Geometry check sheet. Reference: the model listing, model coordinates, mm. Face numbers are marked on the shaded views. A direction names the side the tool comes from. Give positions to 0.01 mm unless a question says otherwise; leave off trailing zeros. Loops run counter-clockwise (first coordinate to the right, second up) from the corner with the lowest first, then second, coordinate; pieces in that order, holes last.
1. Material ranges on L1, parallel to X at y = 2.7, z = -53 (3 decimals); L2, parallel to X at y = 1.35, z = -52; L3, parallel to Z at x = 7, y = 1.5, recorded low to high.
2. Cross-section at D-D, the plane x = -20. Record the cut outline in (y, z).
3. Cross-section at C-C, the plane x = -49. Record the cut outline in (y, z), plus the area to 3 significant figures.
4. Cross-section at A-A, the plane z = -59.5. Record the cut outline in (x, y).
5. Cross-section at B-B, the plane z = -22. Record the cut outline in (x, y), plus the area to 3 significant figures.
6. Tool access check on the marked faces 1 and 2. Record the directions out of +Z, -Z, +X, -X, +Y, -Y that give a thin tool (end or side, any length) a straight path to the whole face; none if there is none.
7. Go/stop test with flat-tipped pins: pin 1 Ø0.6 at (y, z) = (0.5, -8) entering from -X; pin 2 Ø1 at (x, y) = (-86.5, 0.5) entering from -Z; pin 3 Ø1 at (x, z) = (-79.5, -15.5) entering from +Y. Record where each tip stops, or that it passes through.
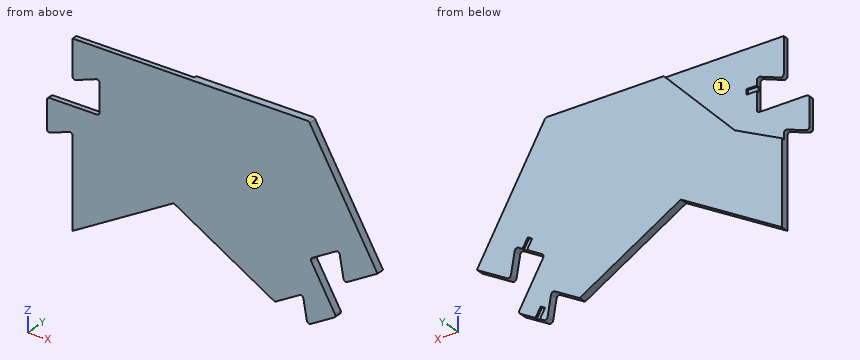
from build123d import *

# Parameters (mm, degrees)
P_IDAT_VYSUNUT_M1_DEPTH  = 3
P_IDAT_VYSUNUT_M2_DEPTH  = 2
ZAOBLIT1_R               = 1
SKICA3_W                 = 4
SKICA3_H                 = 2
ODEBRAT_VYSUNUT_M1_DEPTH = 0.8
ODEBRAT_VYSUNUT_M2_DEPTH = 0.8


with BuildPart() as part:
    # Skica1 → P_idat vysunut_m1 (new body)
    with BuildSketch(Plane(origin=(0, 0, 0), x_dir=(1, 0, 0), z_dir=(0, 1, 0))):
        Polygon((26.667853432, 46.190077074), (13.677472376, 53.690077074), (11.737150801, 42.685966604), (0.392218012, 49.235966604), (10.61747027, 66.946623035), (-0.554257439, 73.396623035), (-2.393036353, 62.968389614), (-13.22114317, 69.22), (-52.538696502, 46.52), (-91.856249834, 69.22), (-91.856249834, 37.22), (-73.49138407, 28.419769911), (-45.928124917, 0), (0, 0), align=None)
    extrude(amount=P_IDAT_VYSUNUT_M1_DEPTH)

    # Skica1_15 → P_idat vysunut_m2 (add)
    with BuildSketch(Plane(origin=(0, 0, 0), x_dir=(1, 0, 0), z_dir=(0, 1, 0))):
        Polygon((13.677472376, 53.690077074), (26.667853432, 46.190077074), (0, 0), (-91.856249834, 0), (-91.856249834, 15), (-81.356249834, 11.17831254), (-81.356249834, 24.27831254), (-101.80675435, 24.27831254), (-101.80675435, 37.17831254), (-91.856249834, 33.55662508), (-91.856249834, 69.22), (-52.538696502, 46.52), (-13.22114317, 69.22), (-2.393036353, 62.968389614), (-0.554257439, 73.396623035), (10.61747027, 66.946623035), (0.392218012, 49.235966604), (11.737150801, 42.685966604), align=None)
    extrude(amount=P_IDAT_VYSUNUT_M2_DEPTH)

    # Zaoblit1
    zaoblit1_edges = [part.edges().sort_by_distance(p)[0] for p in [
        (10.61747027, 1.5, -66.946623035),
        (0.392218012, 1.5, -49.235966604),
        (11.737150801, 1.5, -42.685966604),
        (13.677472376, 1.5, -53.690077074),
        (0, 1.5, 0),
        (-2.393036353, 1.5, -62.968389614),
        (-0.554257439, 1.5, -73.396623035),
        (-91.856249834, 1, -33.55662508),
        (-101.80675435, 1, -37.17831254),
        (-101.80675435, 1, -24.27831254),
        (-81.356249834, 1, -24.27831254),
        (-81.356249834, 1, -11.17831254),
        (-91.856249834, 1, -15),
    ]]
    fillet(zaoblit1_edges, radius=ZAOBLIT1_R)

    # Skica3 → Odebrat vysunut_m1 (cut)
    with BuildSketch(Plane(origin=(0, 2, 0), x_dir=(1, 0, 0), z_dir=(0, 1, 0))):
        with Locations((-79.356249834, 15.42831254)):
            Rectangle(SKICA3_W, SKICA3_H)
    extrude(amount=-ODEBRAT_VYSUNUT_M1_DEPTH, mode=Mode.SUBTRACT)

    # Skica4 → Odebrat vysunut_m2 (cut)
    with BuildSketch(Plane(origin=(0, 3, 0), x_dir=(1, 0, 0), z_dir=(0, 1, 0))):
        Polygon((7.190517431, 45.310966604), (5.190517431, 41.846864989), (6.922568239, 40.846864989), (8.922568239, 44.310966604), align=None)
        Polygon((0.173722583, 68.35752142), (2.173722583, 71.821623035), (3.90577339, 70.821623035), (1.90577339, 67.35752142), align=None)
    extrude(amount=-ODEBRAT_VYSUNUT_M2_DEPTH, mode=Mode.SUBTRACT)


solid = part.part
Result:
1. L1: x = -91.856 to -63.762, -41.315 to 2.565, 13.958 to 14.87
1. L2: x = -91.86 to -62.03, -43.05 to 1.99, 13.38 to 16.6
1. L3: z = -69.04 to -60.68, -45.42 to -12.12
2. outline: (0, -65.31) - (3, -65.31) - (3, 0) - (0, 0) - close
3. outline: (0, -48.56) - (3, -48.56) - (3, -3.17) - (2, -3.17) - (2, 0) - (0, 0) - close
3. area: 143 mm2
4. outline: (-91.86, 0) - (-75.02, 0) - (-75.02, 3) - (-91.86, 3) - close; (-30.06, 0) - (6.32, 0) - (6.32, 3) - (-30.06, 3) - close
5. outline: (-81.36, 0) - (12.7, 0) - (12.7, 3) - (-67.27, 3) - (-67.27, 2) - (-81.36, 2) - close
5. area: 268 mm2
6. face 1: +Z, -X, +Y
6. face 2: +Z, -Z, +X, -X, -Y
7. pin 1: stops at x = -91.86
7. pin 2: stops at z = -66.42
7. pin 3: stops at y = 1.2
